Geometry: see drawing. Coordinates: mm, zero at the bounding-box minimum. A direction names the side the tool comes from. Give positions to 0.01 mm unless a question says otherwise; leave off trailing zeros. Write each loop counter-clockwise with the first axis right and the second up, starting at its lowest first coordinate (ties: lowest second). Pieces come first, ordered by that corner, then holes. Notation, with made-up numbers: (-37.5, 21) -> (21.5, 21) arc R23 cw to (21.5, 39) -> close; hole circle Ø4 at (-39.5, -30.75). An arc over 180 degrees is marked (long way). Use one line per item in the form item = value. Start each with the question number.
(1) Set-up query: the marked faces 4, 5 and 6. Return all of +Z, -Z, +X, -X, +Y, -Y with unobstructed straight access to the full face (end or side cutting, diameter ignored); none if empty.
(2) First-contact query: P1, Ø4, axis at x = 56, y = 17, coming from the +Z side; P2, Ø1, axis at x = 62.5, y = 34, coming from the -Z side; P3, Ø5, axis at y = 40, z = 16.5, coming from the +X side. Flat tips, straight axial feed; report the tip coordinate or a pass-through.
(3) Material intervals for line 1 along Y through (x, z) = (38, 27); line 2 along Z through (x, y) = (38, 7.5); line 3 along Y through (x, z) = (45.5, 32), sorted ascending. Write a range as from..to.
(4) Draft query along Y for the marked faces 1, 2 and 3. Return one class per face: pulls with the +Y half, pulls with the -Y half, needs draft (parallel to the pull), parting line crosses it, or undercut.
(5) Cut plane B-B, the plane z = 31.5. Output: boundary loops of the cut face in (x, y).
(6) Cut plane C-C, the plane y = 41. Output: boundary loops of the cut face in (x, z), and give its area (3 significant figures).
(7) Cut plane D-D, the plane x = 60. Output: boundary loops of the cut face in (y, z), and give its area (3 significant figures).
(8) Cut plane A-A, the plane x = 38.1. Output: boundary loops of the cut face in (y, z), and give its area (3 significant figures).
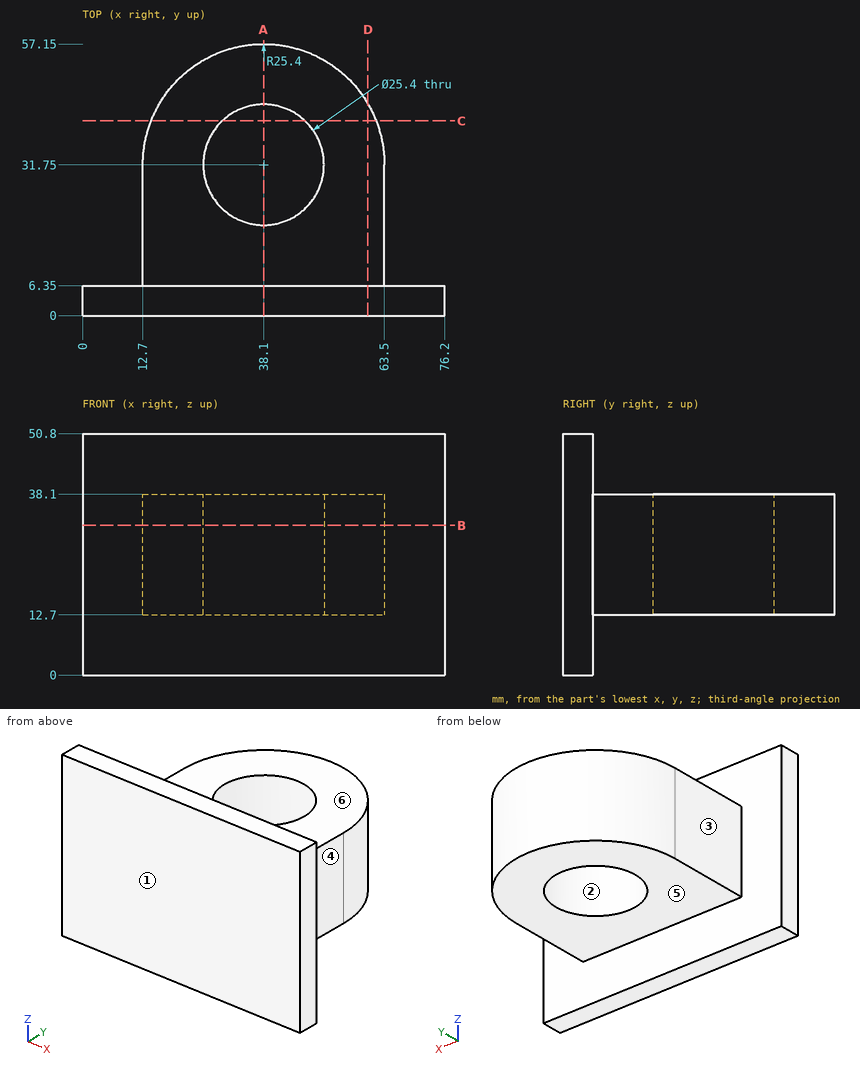
Geometry says:
q1.face_4 = +Z, -Z, +X, +Y
q1.face_5 = -Z, +X, -X, +Y
q1.face_6 = +Z, +X, -X, +Y
q2.P1 = 38.1
q2.P2 = 12.7
q2.P3 = 62.84
q3.line_1 = 0..19.05, 44.45..57.15
q3.line_2 = 12.7..38.1
q3.line_3 = 0..21.43, 42.07..56.05
q4.face_1 = pulls with the -Y half
q4.face_2 = undercut
q4.face_3 = needs draft
q5.outline = (0, 0) -> (76.2, 0) -> (76.2, 6.35) -> (63.5, 6.35) -> (63.5, 31.75) arc R25.4 ccw to (12.7, 31.75) -> (12.7, 6.35) -> (0, 6.35) -> close; hole circle Ø25.4 at (38.1, 31.75)
q6.outline = (14.44, 12.7) -> (29.4, 12.7) -> (29.4, 38.1) -> (14.44, 38.1) -> close; (46.8, 12.7) -> (61.76, 12.7) -> (61.76, 38.1) -> (46.8, 38.1) -> close
q6.area = 760 mm^2
q7.outline = (0, 0) -> (6.35, 0) -> (6.35, 12.7) -> (44.62, 12.7) -> (44.62, 38.1) -> (6.35, 38.1) -> (6.35, 50.8) -> (0, 50.8) -> close
q7.area = 1,290 mm^2
q8.outline = (0, 0) -> (6.35, 0) -> (6.35, 12.7) -> (19.05, 12.7) -> (19.05, 38.1) -> (6.35, 38.1) -> (6.35, 50.8) -> (0, 50.8) -> close; (44.45, 12.7) -> (57.15, 12.7) -> (57.15, 38.1) -> (44.45, 38.1) -> close
q8.area = 968 mm^2
